For this review, take the finished solid that the model builds, in its own axes (mm). A direction names the side the tool comes from. Coordinates: 2 decimals unless noted, no trailing zeros. Loops run counter-clockwise (first coordinate to the right, second up) from the corner with the lowest first, then second, coordinate; pieces in that order, holes last. Notation, with made-up numbers: (18, 75) -> (43, 75) arc R27 ccw to (43, 98) -> close; hole circle Ø6 at (-40, 33). An arc over 180 degrees is marked (long way). Use a Markdown table: item, result.
from build123d import *

# Parameters (mm, degrees)
F1_DEPTH  = 50
F3_DEPTH  = 50
F5_DEPTH  = 5
F7_DEPTH  = 5
F9_DEPTH  = 5
F11_DEPTH = 5
F12_SIZE  = 10
F13_W     = 9
F13_H     = 12
F14_DEPTH = 2
F15_W     = 8
F15_H     = 11.5
F16_DEPTH = 2
F17_W     = 9
F17_H     = 12
F18_DEPTH = 2
F20_W     = 9
F20_H     = 12
F21_DEPTH = 2
F22_W     = 8
F22_H     = 11.5
F23_DEPTH = 2
F24_W     = 9
F24_H     = 12
F25_DEPTH = 2
F26_W     = 8
F26_H     = 11.5
F27_DEPTH = 2
F19_W     = 8
F19_H     = 11.5
F28_DEPTH = 2
F30_DEPTH = 50


with BuildPart() as f1:
    # F0 (on Front) → F1 (new body, symmetric)
    with BuildSketch(Plane.XZ):
        Polygon((-50, -30), (50, -30), (50, 30), (13.3536681533, 30), (10, 33.708491596), (0, 33.708491596), (-10, 33.708491596), (-13.3536681533, 30), (-50, 30), align=None)
    extrude(amount=F1_DEPTH, both=True)

    # F2 (on Right) → F3 (join, symmetric)
    with BuildSketch(Plane.YZ):
        Polygon((10, 33.708491596), (0, 33.708491596), (-10, 33.708491596), (-13.3536681533, 30), (-50, 30), (-50, -30), (0, -30), (50, -30), (50, 30), (13.3536681533, 30), align=None)
    extrude(amount=F3_DEPTH, both=True)

    # F4 (on face) → F5 (cut)
    with BuildSketch(Plane(origin=(-50, 0, 0), x_dir=(0, -1, 0), z_dir=(-1, 0, 0))):
        Polygon((10, 33.708491596), (-10, 33.708491596), (-13.3536681533, 30), (-13.3536681533, -30), (13.3536681533, -30), (13.3536681533, 30), align=None)
    extrude(amount=-F5_DEPTH, mode=Mode.SUBTRACT)

    # F6 (on face) → F7 (cut)
    with BuildSketch(Plane.XZ.offset(50)):
        Polygon((-10, 33.708491596), (-13.3536681533, 30), (-13.3536681533, -30), (13.3536681533, -30), (13.3536681533, 30), (10, 33.708491596), align=None)
    extrude(amount=-F7_DEPTH, mode=Mode.SUBTRACT)

    # F8 (on face) → F9 (cut)
    with BuildSketch(Plane.YZ.offset(50)):
        Polygon((-10, 33.708491596), (-13.3536681533, 30), (-13.3536681533, -30), (13.3536681533, -30), (13.3536681533, 30), (10, 33.708491596), align=None)
    extrude(amount=-F9_DEPTH, mode=Mode.SUBTRACT)

    # F10 (on face) → F11 (cut)
    with BuildSketch(Plane(origin=(0, 50, 0), x_dir=(-1, 0, 0), z_dir=(0, 1, 0))):
        Polygon((-10, 33.708491596), (-13.3536681533, 30), (-13.3536681533, -30), (13.3536681533, -30), (13.3536681533, 30), (10, 33.708491596), align=None)
    extrude(amount=-F11_DEPTH, mode=Mode.SUBTRACT)

    # F12
    f12_edges = [f1.edges().sort_by_distance(p)[0] for p in [
        (50, -50, 0),
        (50, 50, 0),
        (-50, 50, 0),
        (-50, -50, 0),
    ]]
    chamfer(f12_edges, length=F12_SIZE)

    # F13 (on face) → F14 (cut)
    with BuildSketch(Plane(origin=(-45, 45, 0), x_dir=(-0.7071067812, -0.7071067812, 0), z_dir=(-0.7071067812, 0.7071067812, 0))):
        with Locations((0.0210678119, -24)):
            Rectangle(F13_W, F13_H)
    extrude(amount=-F14_DEPTH, mode=Mode.SUBTRACT)

    # F15 (on face) → F16 (join)
    with BuildSketch(Plane(origin=(-43.5857864376, 43.5857864376, 0), x_dir=(-0.7071067812, -0.7071067812, 0), z_dir=(-0.7071067812, 0.7071067812, 0))):
        with Locations((0.0210678119, -24.25)):
            Rectangle(F15_W, F15_H)
    extrude(amount=F16_DEPTH)

    # F17 (on face) → F18 (cut)
    with BuildSketch(Plane(origin=(-45, -45, 0), x_dir=(0.7071067812, -0.7071067812, 0), z_dir=(-0.7071067812, -0.7071067812, 0))):
        with Locations((0.0210678119, -24)):
            Rectangle(F17_W, F17_H)
    extrude(amount=-F18_DEPTH, mode=Mode.SUBTRACT)

    # F20 (on face) → F21 (cut)
    with BuildSketch(Plane(origin=(45, -45, 0), x_dir=(0.7071067812, 0.7071067812, 0), z_dir=(0.7071067812, -0.7071067812, 0))):
        with Locations((0.0210678119, -24)):
            Rectangle(F20_W, F20_H)
    extrude(amount=-F21_DEPTH, mode=Mode.SUBTRACT)

    # F22 (on face) → F23 (join)
    with BuildSketch(Plane(origin=(43.5857864376, -43.5857864376, 0), x_dir=(0.7071067812, 0.7071067812, 0), z_dir=(0.7071067812, -0.7071067812, 0))):
        with Locations((0.0210678119, -24.25)):
            Rectangle(F22_W, F22_H)
    extrude(amount=F23_DEPTH)

    # F24 (on face) → F25 (cut)
    with BuildSketch(Plane(origin=(45, 45, 0), x_dir=(-0.7071067812, 0.7071067812, 0), z_dir=(0.7071067812, 0.7071067812, 0))):
        with Locations((0.0210678119, -24)):
            Rectangle(F24_W, F24_H)
    extrude(amount=-F25_DEPTH, mode=Mode.SUBTRACT)

    # F26 (on face) → F27 (join)
    with BuildSketch(Plane(origin=(43.5857864376, 43.5857864376, 0), x_dir=(-0.7071067812, 0.7071067812, 0), z_dir=(0.7071067812, 0.7071067812, 0))):
        with Locations((0.0210678119, -24.25)):
            Rectangle(F26_W, F26_H)
    extrude(amount=F27_DEPTH)

    # F19 (on face) → F28 (join)
    with BuildSketch(Plane(origin=(-43.5857864376, -43.5857864376, 0), x_dir=(0.7071067812, -0.7071067812, 0), z_dir=(-0.7071067812, -0.7071067812, 0))):
        with Locations((0.0210678119, -24.25)):
            Rectangle(F19_W, F19_H)
    extrude(amount=F28_DEPTH)

    # F29 (on face) → F30 (cut)
    with BuildSketch(Plane.XY.offset(33.708491596)):
        Polygon((-44, 9), (-44, -9), (-9, -9), (-9, -44), (9, -44), (9, -9), (44, -9), (44, 9), (9, 9), (9, 44), (-9, 44), (-9, 9), align=None)
    extrude(amount=-F30_DEPTH, mode=Mode.SUBTRACT)


solid = f1.part
(1) Mouldability with a two-part tool opening along X and no side actions: class faces 6 (the face through (-45, 45, -24)), 7 (the face through (-48, -13.354, 0)), 8 (the face through (-13.354, 48, 0)) as pulls with the +X half, pulls with the -X half, needs draft (parallel to the pull), parting line crosses it, or undercut.
Found:
| item | result |
|---|---|
| face 6 | pulls with the -X half |
| face 7 | needs draft |
| face 8 | undercut |
(2) Take a section at A-A on y = -22.5. Write out the cut boundary in (x, z).
Found:
| item | result |
|---|---|
| outline | (-50, -30) -> (50, -30) -> (50, 30) -> (13.35, 30) -> (10, 33.71) -> (9, 33.71) -> (9, -16.29) -> (-9, -16.29) -> (-9, 33.71) -> (-10, 33.71) -> (-13.35, 30) -> (-50, 30) -> close |
(3) For faces 1 (the face through (-9, -26, 9)), 2 (the face through (-11.653, -27.745, 31.88)), 3 (the face through (11.7, -27.74, 31.83)), 4 (the face through (45, -45, 0)), 5 (the face through (-13.354, -48, 0)), list the 3-axis set-ups (+Z, -Z, +X, -X, +Y, -Y) from which the entire face can be reached by the end or side of a thin tool; tool diameter is ignored.
Found:
| item | result |
|---|---|
| face 1 | +Z |
| face 2 | +Z, -X, -Y |
| face 3 | +Z, +X, -Y |
| face 4 | +Z, -Z, +X, -Y |
| face 5 | +Z, -Z, -Y |
(4) For line 1 along X through (y, z) = (13, 24); line 2 along Y through (x, z) = (-33, 17), list the stretches that pass through material, from the lowest coordinate up.
Found:
| item | result |
|---|---|
| line 1 | x = -45 to -9, 9 to 45 |
| line 2 | y = -50 to -9, 9 to 50 |
(5) For pin 1 Ø9 at (y, z) = (1, 6.5) entering from +X; pin 2 Ø8 at (x, y) = (-42.5, 46) entering from +Z; pin 3 Ø3 at (x, z) = (-7.5, -5) entering from +Y, all flat-tipped, find the tip position at first contact; note any pin that passes through.
Found:
| item | result |
|---|---|
| pin 1 | stops at x = 45 |
| pin 2 | stops at z = 30 |
| pin 3 | stops at y = 45 |
